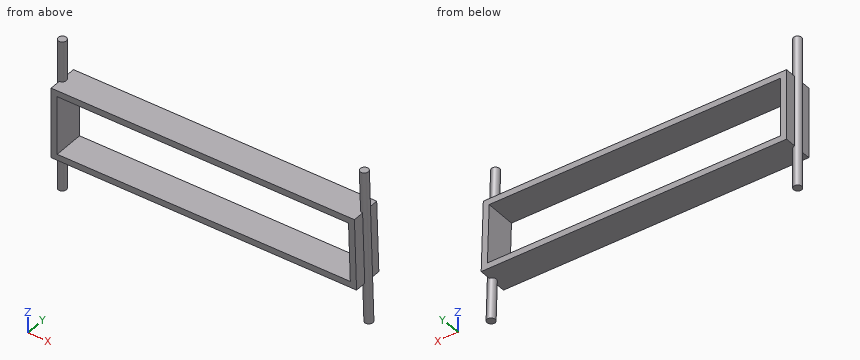
```python
from build123d import *

# Parameters (mm, degrees)
BOSS_EXTRUDE1_DEPTH = 38.1
SKETCH2_R           = 5.08
BOSS_EXTRUDE2_DEPTH = 95.25


with BuildPart() as part:
    # Sketch1 → Boss-Extrude1 (new body)
    with BuildSketch(Plane(origin=(0, 0, 0), x_dir=(1, 0, 0), z_dir=(0, 1, 0))):
        Polygon((-323.578651022, -44.335687139), (57.378484067, -50.050687139), (60.045184013, 38.809307861), (-323.578651022, 44.564312861), align=None)
        Polygon((-315.958651022, -36.829142605), (49.987084067, -42.318946269), (52.196584013, 31.306192713), (-315.958651022, 36.829142605), align=None, mode=Mode.SUBTRACT)
    extrude(amount=-BOSS_EXTRUDE1_DEPTH)

    # Sketch2 → Boss-Extrude2 (add, symmetric)
    with BuildSketch(Plane.XY):
        with Locations((-323.578651022, -19.05)):
            Circle(SKETCH2_R)
    boss_extrude2 = extrude(amount=BOSS_EXTRUDE2_DEPTH, both=True)

    # Mirror1: Boss-Extrude2 across plane
    add(boss_extrude2.mirror(Plane(origin=(-132.362317794, 0, -1.985658166), x_dir=(-0.015, 0, 0.999887494), z_dir=(0.999887494, 0, 0.015))))


solid = part.part
```
Here's how the part is built. I have some questions about the finished solid (model axes, mm). Round coordinates to 2 decimals unless told otherwise and drop trailing zeros. Write each loop counter-clockwise with the first axis right and the second up, starting at its lowest first coordinate (ties: lowest second). Pieces come first, ordered by that corner, then holes.
Q1. If we section it at A-A on y = -33: Write out the boundary of the cut face in (x, z), plus the area to 3 significant figures.
Q2. If we section it at B-B on x = -84: Write out the boundary of the cut face in (y, z), plus the area to 3 significant figures.
Q3. Please list where these lines run through material, in increasing order: probe 1 along Z at (x, y) = (-152.5, -15.5); probe 2 along Z at (x, y) = (-203, -27.5); probe 3 along X at (y, z) = (-15.5, 67.5).
Q4. Will these pins go through, and if not, where does the flat tip stop? P1, Ø3, axis at y = -21, z = 49, coming from the -X side; P2, Ø11, axis at x = -322.5, y = -21, coming from the +Z side; P3, Ø11, axis at y = -9, z = -18.5, coming from the -X side.
Answer below:
1. outline: (-323.58, -44.56) - (60.05, -38.81) - (57.38, 50.05) - (-323.58, 44.34) - close; hole (-315.96, -36.83) - (52.2, -31.31) - (49.99, 42.32) - (-315.96, 36.83) - close
1. area: 6,950 mm2
2. outline: (-38.1, -40.97) - (0, -40.97) - (0, -33.35) - (-38.1, -33.35) - close; (-38.1, 40.31) - (0, 40.31) - (0, 47.93) - (-38.1, 47.93) - close
2. area: 581 mm2
3. probe 1: z = -42 to -34.38, 39.28 to 46.9
3. probe 2: z = -42.76 to -35.13, 38.52 to 46.14
3. probe 3: x = -327.21 to -319.94, 53.22 to 60.49
4. P1: stops at x = -328.64
4. P2: stops at z = 95.25
4. P3: stops at x = -325.84
